Verification items for the finished model (mm, model axes). A direction names the side the tool comes from. Give positions to 0.01 mm unless a question says otherwise; leave off trailing zeros. Loops run counter-clockwise (first coordinate to the right, second up) from the corner with the lowest first, then second, coordinate; pieces in that order, holes last. Notation, with made-up numbers: (58, 31) -> (91, 31) arc R22 cw to (91, 63) -> close; hole circle Ø4 at (0, 48.5). An arc over 180 degrees is marked (long way). Use one line per item in the form item = value. Start each with the question number.
from build123d import *

# Parameters (mm, degrees)
F1_DEPTH = 50
F4_DEPTH = 60
F5_R     = 26
F6_DEPTH = 15
F10_SIZE = 5
F11_SIZE = 5
F12_SIZE = 5


with BuildPart() as f1:
    # F0 (on Front) → F1 (new body)
    with BuildSketch(Plane.XZ):
        with BuildLine():
            Line((111, 76), (0, 76))
            ThreePointArc((0, 76), (-76, 0), (0, -76))
            Line((0, -76), (111, -76))
            ThreePointArc((111, -76), (187, 0), (111, 76))
        make_face()
    extrude(amount=F1_DEPTH)

    # F3 (on offset) + F1_face (on face) → F4 (cut)
    with BuildSketch(Plane.XZ.offset(19)):
        with BuildLine():
            Line((111, 64), (0, 64))
            ThreePointArc((0, 64), (-64, 0), (0, -64))
            Line((0, -64), (111, -64))
            ThreePointArc((111, -64), (175, 0), (111, 64))
        make_face()
    with BuildSketch(Plane(origin=(55.5, -50, 0), x_dir=(1, 0, 0), z_dir=(0, -1, 0))):
        with BuildLine():
            Line((55.5, 76), (-55.5, 76))
            ThreePointArc((-55.5, 76), (-131.5, 0), (-55.5, -76))
            Line((-55.5, -76), (55.5, -76))
            ThreePointArc((55.5, -76), (131.5, 0), (55.5, 76))
        make_face()
    extrude(amount=F4_DEPTH, mode=Mode.SUBTRACT)

    # F5 (on offset) → F6 (cut)
    with BuildSketch(Plane.XZ.offset(19)):
        Circle(F5_R)
    extrude(amount=-F6_DEPTH, mode=Mode.SUBTRACT)

    # F8 (on offset) → F9 (revolve, cut)
    with BuildSketch(Plane.YZ.offset(111)):
        Polygon((0, 0), (0, 11), (-2, 11), (-2, 18.5), (-7, 18.5), (-7, 23.5), (-19, 23.5), (-19, 0), align=None)
    revolve(axis=Axis((111, -9.5, 0), (0, 1, 0)), mode=Mode.SUBTRACT)

    # F10
    f10_edges = [f1.edges().sort_by_distance(p)[0] for p in [
        (55.5, 0, 76),
        (187, 0, 0),
        (-76, 0, 0),
        (55.5, 0, -76),
    ]]
    chamfer(f10_edges, length=F10_SIZE)

    # F11
    f11_edges = [f1.edges().sort_by_distance(p)[0] for p in [
        (55.5, -50, 76),
        (-76, -50, 0),
        (187, -50, 0),
        (55.5, -50, -76),
    ]]
    chamfer(f11_edges, length=F11_SIZE)

    # F12
    f12_edges = [f1.edges().sort_by_distance(p)[0] for p in [
        (55.5, -50, 64),
        (-64, -50, 0),
        (55.5, -50, -64),
        (175, -50, 0),
    ]]
    chamfer(f12_edges, length=F12_SIZE)


solid = f1.part
Item 1: Tool access check on faces 1 (the flat face through (56, -25, 76)), 2 (the flat face through (56, -32, 64)). Record the directions out of +Z, -Z, +X, -X, +Y, -Y that give a thin tool (end or side, any length) a straight path to the whole face; none if there is none.
Item 2: Sectioned sample at D-D, the plane y = -13. Enter the section's corners in (x, z), and give its area (3 significant figures).
Item 3: Sectioned sample at B-B, the plane y = -27. Enter the section's corners in (x, z).
Item 4: Material ranges on line 1 (Z direction, x = 0, y = -14.5); line 2 (X direction, y = -17.5, z = 7); line 3 (Y direction, x = 71.5, z = -31), recorded low to high.
Item 5: Gauge pin test, flat ends, axial feed: pin 1 Ø8 at (x, y) = (-29, -6.5) entering from +Z; pin 2 Ø5 at (x, y) = (-45.5, -41.5) entering from -Z; pin 3 Ø12 at (x, z) = (128.5, 23.5) entering from -Y. Record the tip position at first contact, or that the pin passes through.
Item 6: Sectioned sample at C-C, the plane x = 31.5. Enter the section's corners in (y, z), and give its area (3 significant figures).
Outcome:
q1.face_1 = +Z, +X, -X, +Y, -Y
q1.face_2 = -Y
q2.outline = (0, -76) -> (111, -76) arc R76 ccw to (111, 76) -> (0, 76) arc R76 ccw to start; hole circle Ø52 at (0, 0); hole circle Ø47 at (111, 0)
q2.area = 31,200 mm^2
q3.outline = (0, -76) -> (111, -76) arc R76 ccw to (111, 76) -> (0, 76) arc R76 ccw to start; hole (0, -64) -> (111, -64) arc R64 ccw to (111, 64) -> (0, 64) arc R64 ccw to start
q4.line_1 = -76 to -26, 26 to 76
q4.line_2 = -75.68 to -25.04, 25.04 to 88.57, 133.43 to 186.68
q4.line_3 = -19 to 0
q5.pin_1 = 71.77
q5.pin_2 = -62.67
q5.pin_3 = -19
q6.outline = (-50, -71) -> (-45, -76) -> (-5, -76) -> (0, -71) -> (0, 71) -> (-5, 76) -> (-45, 76) -> (-50, 71) -> (-50, 69) -> (-45, 64) -> (-19, 64) -> (-19, -64) -> (-45, -64) -> (-50, -69) -> close
q6.area = 3,560 mm^2
